Could you check a few things on this model? Use its own coordinates, in mm. A direction names the side the tool comes from. Give positions to 0.01 mm unless a question says otherwise; leave off trailing zeros. Loops run counter-clockwise (first coordinate to the right, second up) from the corner with the lowest first, then second, coordinate; pieces in that order, holes last. Notation, with made-up numbers: (82, 65) - (118, 65) arc R14 cw to (118, 71) - close; hole circle Ø8 at (70, 88). An arc over 180 degrees is marked (long way). Use CSV: the item, a comma, the result in double quotes.
from build123d import *

# Parameters (mm, degrees)
SKETCH1_R           = 0.525
BOSS_EXTRUDE1_DEPTH = 1.5
BOSS_EXTRUDE2_DEPTH = 4
SKETCH4_W           = 6
SKETCH4_H           = 16
CHAMFER1_SIZE       = 1


with BuildPart() as part:
    # Sketch1 → Boss-Extrude1 (new body)
    with BuildSketch(Plane.XY):
        Polygon((-20, 17), (-17, 20), (17, 20), (20, 17), (20, -17), (17, -20), (-17, -20), (-20, -17), align=None)
        with Locations((-17, 17)):
            Circle(SKETCH1_R, mode=Mode.SUBTRACT)
        with Locations((17, 17)):
            Circle(SKETCH1_R, mode=Mode.SUBTRACT)
        with Locations((17, -17)):
            Circle(SKETCH1_R, mode=Mode.SUBTRACT)
        with Locations((-17, -17)):
            Circle(SKETCH1_R, mode=Mode.SUBTRACT)
        with Locations((10, 0)):
            Circle(SKETCH1_R, mode=Mode.SUBTRACT)
        with Locations((-10, 0)):
            Circle(SKETCH1_R, mode=Mode.SUBTRACT)
    extrude(amount=BOSS_EXTRUDE1_DEPTH)

    # Sketch3 → Boss-Extrude2 (add)
    with BuildSketch(Plane.XY.offset(1.5)):
        with BuildLine():
            Line((-6, -7), (6, -7))
            ThreePointArc((6, -7), (6.707106781, -6.707106781), (7, -6))
            Line((7, -6), (7, 6))
            ThreePointArc((7, 6), (6.707106781, 6.707106781), (6, 7))
            Line((6, 7), (-6, 7))
            ThreePointArc((-6, 7), (-6.707106781, 6.707106781), (-7, 6))
            Line((-7, 6), (-7, -6))
            ThreePointArc((-7, -6), (-6.707106781, -6.707106781), (-6, -7))
        make_face()
    extrude(amount=BOSS_EXTRUDE2_DEPTH)

    # Sketch4 → Revolve1 (revolve)
    with BuildSketch(Plane(origin=(0, 0, 0), x_dir=(1, 0, 0), z_dir=(0, 1, 0)), mode=Mode.PRIVATE) as revolve1_sk:
        with Locations((-3, -13.5)):
            Rectangle(SKETCH4_W, SKETCH4_H)
    revolve(revolve1_sk.sketch.rotate(Axis((0, 0, 1000), (0, 0, -1)), 180), axis=Axis((0, 0, 1000), (0, 0, -1)))

    # Chamfer1
    chamfer1_edges = [part.edges().sort_by_distance(p)[0] for p in [
        (-6, 0, 21.5),
    ]]
    chamfer(chamfer1_edges, length=CHAMFER1_SIZE)


solid = part.part
1) Suppose I cut it at B-B (x = 10). Please give me the cut outline in (y, z) (3 decimals), plus the area to 3 significant figures.
Answer below:
outline,"(-20, 0) - (-0.525, 0) - (-0.525, 1.5) - (-20, 1.5) - close; (0.525, 0) - (20, 0) - (20, 1.5) - (0.525, 1.5) - close"
area,"58.4 mm2"
2) Which directions (+Z, -Z, +X, -X, +Y, -Y) give clear straight access to the entire face, cutting with the end or side of a thin tool? Please do faces 4 (the cylindrical face through (6.715, 6.699, 3.472)), 5 (the cylindrical face through (6.699, -6.715, 3.472)), 6 (the flat face through (7, 0, 3)), 7 (the flat face through (-9, 0, 1.5)), 8 (the flat face through (20, 0, 1)).
Answer below:
face 4,"+Z, +X, +Y"
face 5,"+Z, +X, -Y"
face 6,"+Z, +X, +Y, -Y"
face 7,"+Z"
face 8,"+Z, -Z, +X, +Y, -Y"
3) Suppose I cut it at D-D (x = 0). Please give me the cut outline in (y, z).
Answer below:
outline,"(-20, 0) - (20, 0) - (20, 1.5) - (7, 1.5) - (7, 5.5) - (6, 5.5) - (6, 20.5) - (5, 21.5) - (-5, 21.5) - (-6, 20.5) - (-6, 5.5) - (-7, 5.5) - (-7, 1.5) - (-20, 1.5) - close"
4) We'd pull the mould along X, two halves only. Please class faces 1 (the cylindrical face through (-17.114, -17.513, 0.74)), 2 (the flat face through (-7, 0, 3)), 3 (the flat face through (0, 7, 3)): +X half, -X half, draft (parallel to the pull), parting line (faces both ways), or undercut.
Answer below:
face 1,"undercut"
face 2,"-X half"
face 3,"draft"
5) I'm going to push flat-ended pins straight in: P1, Ø4, axis at x = -14, y = -15.5, coming from the -Z side; P2, Ø3, axis at x = 13, y = -11, coming from the +Z side; P3, Ø1, axis at x = 5, z = 15, coming from the +Y side; P4, Ø1.2, axis at y = 0, z = 2.5, coming from the +X side. Where does each tip first touch, or does it pass through?
Answer below:
P1,"stops at z = 0"
P2,"stops at z = 1.5"
P3,"stops at y = 3.97"
P4,"stops at x = 7"
6) Suppose I cut it at A-A (y = 0). Please give me the cut outline in (x, z) (3 decimals).
Answer below:
outline,"(-20, 0) - (-10.525, 0) - (-10.525, 1.5) - (-20, 1.5) - close; (-9.475, 0) - (9.475, 0) - (9.475, 1.5) - (7, 1.5) - (7, 5.5) - (6, 5.5) - (6, 20.5) - (5, 21.5) - (-5, 21.5) - (-6, 20.5) - (-6, 5.5) - (-7, 5.5) - (-7, 1.5) - (-9.475, 1.5) - close; (10.525, 0) - (20, 0) - (20, 1.5) - (10.525, 1.5) - close"
7) Suppose I cut it at C-C (z = 3.25). Please give me the cut outline in (x, y).
Answer below:
outline,"(-7, -6) arc R1 ccw to (-6, -7) - (6, -7) arc R1 ccw to (7, -6) - (7, 6) arc R1 ccw to (6, 7) - (-6, 7) arc R1 ccw to (-7, 6) - close"
8) I need wall thicknesses on line 1 along Y through (x, z) = (-17, 0.9) (3 decimals); line 2 along Y through (x, z) = (10, 0.3) (3 decimals); line 3 along Y through (x, z) = (-3, 4.25). Which ranges of each line are inside material? Lowest first, please.
Answer below:
line 1,"y = -20 to -17.525, -16.475 to 16.475, 17.525 to 20"
line 2,"y = -20 to -0.525, 0.525 to 20"
line 3,"y = -7 to 7"
